Geometry check sheet. Reference: the model listing, model coordinates, mm. A direction names the side the tool comes from. Round coordinates to 2 decimals unless told otherwise and drop trailing zeros. Write each loop counter-clockwise with the first axis right and the second up, starting at its lowest first coordinate (ties: lowest second). Pieces come first, ordered by that corner, then holes. Notation, with made-up numbers: M -39.75,21.5 L -33.75,21.5 A19 cw -33.75,55.5 Z; hole C 42.25,29 d2. An arc over 180 degrees is marked long. Answer as CSV lines item,"result". Start each with the question number.
```python
from build123d import *

# Parameters (mm, degrees)
BOSS_EXTRUDE1_DEPTH = 5
FILLET1_R           = 10
FILLET2_R           = 3
SKETCH2_W           = 30
SKETCH2_H           = 13
CUT_EXTRUDE1_DEPTH  = 358.217020871
SKETCH3_R           = 6.5
CUT_EXTRUDE2_DEPTH  = 358.217020871
CUT_EXTRUDE3_DEPTH  = 358.217020871


with BuildPart() as part:
    # Sketch1 → Boss-Extrude1 (new, symmetric)
    with BuildSketch(Plane(origin=(0, 0, 0), x_dir=(0, 0, -1), z_dir=(1, 0, 0))):
        with BuildLine():
            Line((30, 0), (0, 0))
            Line((0, 0), (0, -50))
            Line((0, -50), (-5, -70))
            Line((-5, -70), (-17, -70))
            Line((-17, -70), (-17, -64))
            ThreePointArc((-17, -64), (-30, -51), (-43, -64))
            Line((-43, -64), (-43, -70))
            Line((-43, -70), (-60, -70))
            Line((-60, -70), (-60, -20))
            Line((-60, -20), (-30, 352))
            Line((-30, 352), (30, 352))
            Line((30, 352), (30, 0))
        make_face()
    extrude(amount=BOSS_EXTRUDE1_DEPTH, both=True)

    # Fillet1
    # the kernel refuses this fillet: 10 mm, written as the material it takes off along each edge
    with BuildSketch(Plane(origin=(8.07764064, -50, 0), x_dir=(0, -0.9701425001453321, 0.24253562503633222), z_dir=(-1, 0, 0))) as fillet1_piece_1:
        with BuildLine():
            CenterArc((FILLET1_R * 0.123105625618, FILLET1_R), FILLET1_R, 255.963756532, 14.036243468)
            Line((-FILLET1_R * 0.119429999419, FILLET1_R * 0.0298574998547), (0, 0))
            Line((0, 0), (FILLET1_R * 0.123105625618, 0))
        make_face()
    extrude(amount=16.155281281, mode=Mode.SUBTRACT)
    with BuildSketch(Plane(origin=(24.51941016, -70, 5), x_dir=(0, 0, 1), z_dir=(-1, 0, 0))) as fillet1_piece_2:
        with BuildLine():
            CenterArc((FILLET1_R * 0.780776406404, FILLET1_R), FILLET1_R, 194.036243468, 75.963756532)
            Line((-FILLET1_R * 0.189366093741, FILLET1_R * 0.757464374964), (0, 0))
            Line((0, 0), (FILLET1_R * 0.780776406404, 0))
        make_face()
    extrude(amount=49.03882032, mode=Mode.SUBTRACT)
    with BuildSketch(Plane(origin=(30, -70, 60), x_dir=(0, 1, 0), z_dir=(-1, 0, 0))) as fillet1_piece_3:
        with BuildLine():
            CenterArc((FILLET1_R, FILLET1_R), FILLET1_R, 180, 90)
            Line((0, FILLET1_R), (0, 0))
            Line((0, 0), (FILLET1_R, 0))
        make_face()
    extrude(amount=60, mode=Mode.SUBTRACT)
    with BuildSketch(Plane(origin=(6.006430802, -20, 60), x_dir=(0, 0.9967639550118461, -0.08038418992029778), z_dir=(-1, 0, 0))) as fillet1_piece_4:
        with BuildLine():
            CenterArc((FILLET1_R * 0.0402572320672, FILLET1_R), FILLET1_R, 265.389350681, 4.610649319)
            Line((-FILLET1_R * 0.0401269578531, FILLET1_R * 0.00323604498815), (0, 0))
            Line((0, 0), (FILLET1_R * 0.0402572320672, 0))
        make_face()
    extrude(amount=12.012861603, mode=Mode.SUBTRACT)
    with BuildSketch(Plane(origin=(-28.065034742, 352, 30), x_dir=(0, 0, -1), z_dir=(1, 0, 0))) as fillet1_piece_5:
        with BuildLine():
            CenterArc((FILLET1_R * 0.922601389683, -FILLET1_R), FILLET1_R, 90, 85.389350681)
            Line((-FILLET1_R * 0.074162565329, -FILLET1_R * 0.91961581008), (0, 0))
            Line((0, 0), (FILLET1_R * 0.922601389683, 0))
        make_face()
    extrude(amount=56.130069484, mode=Mode.SUBTRACT)

    # Fillet2
    fillet2_edges = [part.edges().sort_by_distance(p)[0] for p in [
        (0, -70, 17),
        (0, -70, 43),
    ]]
    fillet(fillet2_edges, radius=FILLET2_R)

    # Sketch2 → Cut-Extrude1 (cut, through all)
    with BuildSketch(Plane(origin=(5, 0, 0), x_dir=(0, 0, -1), z_dir=(1, 0, 0))):
        with Locations((15, 345.5)):
            Rectangle(SKETCH2_W, SKETCH2_H)
    extrude(amount=-CUT_EXTRUDE1_DEPTH, mode=Mode.SUBTRACT)

    # Sketch3 → Cut-Extrude2 (cut, through all)
    with BuildSketch(Plane(origin=(5, 0, 0), x_dir=(0, 0, -1), z_dir=(1, 0, 0))):
        with Locations((-5, 224)):
            Circle(SKETCH3_R)
    extrude(amount=-CUT_EXTRUDE2_DEPTH, mode=Mode.SUBTRACT)

    # Sketch4 → Cut-Extrude3 (cut, through all)
    with BuildSketch(Plane(origin=(5, 0, 0), x_dir=(0, 0, -1), z_dir=(1, 0, 0))):
        with BuildLine():
            ThreePointArc((5.771557213, 229.410506159), (-4.437877767, 230.475648122), (-14.678140573, 231.185653536))
            ThreePointArc((-14.678140573, 231.185653536), (-21.506336405, 225.031326466), (-15.352009335, 218.203130634))
            ThreePointArc((-15.352009335, 218.203130634), (-5.562122233, 217.524351878), (4.198292879, 216.506055789))
            ThreePointArc((4.198292879, 216.506055789), (11.437150231, 222.171648807), (5.771557213, 229.410506159))
        make_face()
    extrude(amount=-CUT_EXTRUDE3_DEPTH, mode=Mode.SUBTRACT)


solid = part.part
```
1) Scan lines: line 1 (Y direction, x = 3.5, z = -21); line 2 (Y direction, x = 1, z = 8); line 3 (Z direction, x = 4.25, y = 225.5). Record each from-to range of solid material in increasing order. Write a range as from..to.
2) Access from +Z, -Z, +X, -X, +Y, -Y to the whole of each face (thin tool, end or side, straight path). Record for faces 4 (the flat face through (0, 345, 0)), 5 (the flat face through (0, 0, -15)), 6 (the cylindrical face through (0.07, 230.463, 4.295)).
3) Mould release check, pull along Z, two halves, no side actions. Record for faces 1 (the flat face through (0.07, 159.07, 45.56)), 2 (the flat face through (0, 339, -15)), 3 (the cylindrical face through (0.07, 222.03, -11.42)): released by +Z, released by -Z, zero draft, split by the parting line, or undercut.
4) Section check A-A, the plane z = -24. Record the cut outline in (x, y), plus the area to 3 significant figures.
5) Go/stop test with flat-tipped pins: pin 1 (0.9 mm diameter, centred on x = -1.5, y = -66, fed in from +Z); pin 2 (1.5 mm diameter, centred on x = 0, y = 61, fed in from +Z); pin 3 (5 mm diameter, centred on x = 2.5, z = -16, fed in from -Y). Record where each tip stops, or that it passes through.
6) Section check B-B, the plane y = 270. Record the cut outline in (x, z).
Results:
1,line 1,"y = 0..339"
1,line 2,"y = -68.77..217.73, 230.76..352"
1,line 3,"z = -30..-10.97, 21.46..40.2"
2,face 4,"-Z, +X, -X, +Y"
2,face 5,"-Z, +X, -X, -Y"
2,face 6,"+X, -X"
3,face 1,"released by +Z"
3,face 2,"zero draft"
3,face 3,"undercut"
4,outline,"M -5,0 L 5,0 L 5,339 L -5,339 Z"
4,area,"3,390 mm^2"
5,pin 1,"stops at z = 58.32"
5,pin 2,"stops at z = 53.53"
5,pin 3,"stops at y = 0"
6,outline,"M -5,-30 L 5,-30 L 5,36.61 L -5,36.61 Z"
